```python
from build123d import *

# Parameters (mm, degrees)
F0_W     = 50
F0_H     = 17
F1_DEPTH = 17
F2_R     = 3
F3_DEPTH = 50.1
F4_R     = 2
F5_DEPTH = 4


with BuildPart() as f1:
    # F0 (on Front) → F1 (new body)
    with BuildSketch(Plane.XZ):
        with Locations((-22.598265, 1.11262)):
            Rectangle(F0_W, F0_H)
    extrude(amount=F1_DEPTH)

    # F2 (on face) → F3 (cut)
    with BuildSketch(Plane.YZ.offset(2.401735)):
        with Locations((-8.5, 0)):
            Circle(F2_R)
    extrude(amount=-F3_DEPTH, mode=Mode.SUBTRACT)

    # F4 (on face) → F5 (cut)
    with BuildSketch(Plane.XY.offset(9.61262)):
        with Locations((-22.598265, -8.5)):
            Circle(F4_R)
    extrude(amount=-F5_DEPTH, mode=Mode.SUBTRACT)


solid = f1.part
```
CAD build for the part. Positions are in the model's coordinates, mm. A direction names the side the tool comes from. Coordinates: 2 decimals unless noted, no trailing zeros. Order: outer loops, then holes, each group sorted by start corner. A loop starts at its lowest first (then second) coordinate and runs counter-clockwise, first axis right, second up.
(1) Saw through at C-C, the plane x = -7. Write the cut outline in (y, z).
Solution:
outline: (-17, -7.39) - (0, -7.39) - (0, 9.61) - (-17, 9.61) - close; hole circle Ø6 at (-8.5, 0)
(2) Saw through at D-D, the plane x = -24. Write the cut outline in (y, z), and give its area (3 significant figures).
Solution:
outline: (-17, -7.39) - (0, -7.39) - (0, 9.61) - (-7.07, 9.61) - (-7.07, 5.61) - (-9.93, 5.61) - (-9.93, 9.61) - (-17, 9.61) - close; hole circle Ø6 at (-8.5, 0)
area: 249 mm2
(3) Pin check, flat tips, straight feed: pin 1 Ø6 at (y, z) = (-7.5, 0.5) entering from -X; pin 2 Ø3 at (x, y) = (-22.6, -8.5) entering from +Z. Stop position of each tip, or through.
Solution:
pin 1: stops at x = -47.6
pin 2: stops at z = 5.61
(4) Mould opens along X. For faces 1 (the face through (-23, -8, 5.613)), 2 (the face through (-47.598, -6, 3)), 3 (the face through (-23, -17, 1)) say: released by +X, released by -X, zero draft, split by the parting line, or undercut.
Solution:
face 1: undercut
face 2: released by -X
face 3: zero draft
(5) Drill centre lines: L1, parallel to Z at x = -16, y = -8.5; L2, parallel to Z at x = -9, y = -9.75; L3, parallel to Y at x = -9.5, z = -2.75. Where is each one in solid material? Low to high.
Solution:
L1: z = -7.39 to -3, 3 to 9.61
L2: z = -7.39 to -2.73, 2.73 to 9.61
L3: y = -17 to -9.7, -7.3 to 0
(6) Saw through at A-A, the plane z = 1.75. Write the cut outline in (x, y).
Solution:
outline: (-47.6, -17) - (2.4, -17) - (2.4, -10.94) - (-47.6, -10.94) - close; (-47.6, -6.06) - (2.4, -6.06) - (2.4, 0) - (-47.6, 0) - close
(7) Which spindle directions (+Z, -Z, +X, -X, +Y, -Y) get a long thin tool onto all of the face, cutting with end or side? Do faces 4 (the face through (-23, 0, 1)), 5 (the face through (-20.69, -7.9, 7.64)). Say none if no direction does.
Solution:
face 4: +Z, -Z, +X, -X, +Y
face 5: +Z
(8) Saw through at B-B, the plane y = -8.5. Write the cut outline in (x, z), and give its area (3 significant figures).
Solution:
outline: (-47.6, -7.39) - (2.4, -7.39) - (2.4, -3) - (-47.6, -3) - close; (-47.6, 3) - (2.4, 3) - (2.4, 9.61) - (-20.6, 9.61) - (-20.6, 5.61) - (-24.6, 5.61) - (-24.6, 9.61) - (-47.6, 9.61) - close
area: 534 mm2
